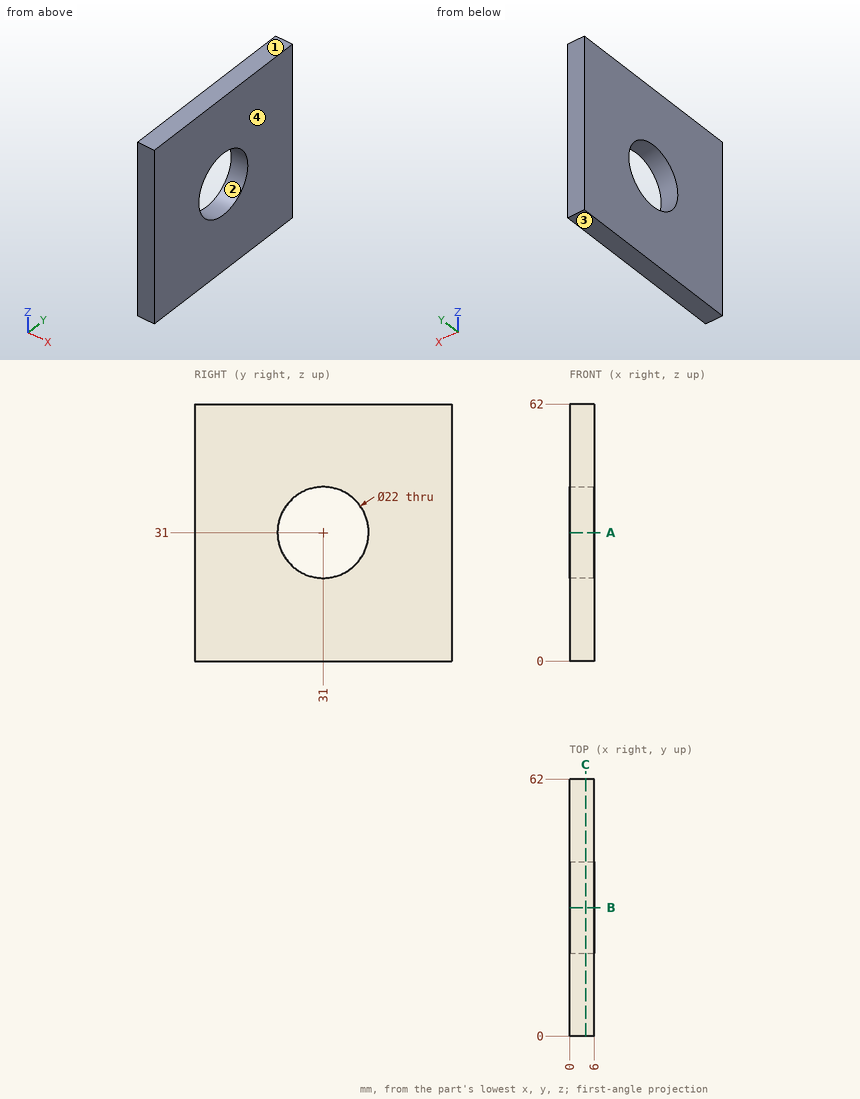
Check sheet for the drawn part. Datum: minimum x, y, z corner. Units: mm. Round coordinates to 2 decimals unless told otherwise and drop trailing zeros. Order: outer loops, then holes, each group sorted by start corner. A loop starts at its lowest first (then second) coordinate and runs counter-clockwise, first axis right, second up.
1) Section check A-A (z = 31). Record the boundary of the cut face in (x, y).
2) Section check C-C (x = 3.85). Record the boundary of the cut face in (y, z).
3) Mould release check, pull along Z, two halves, no side actions. Record for the marked faces 1, 2, 3 and 4: +Z half, -Z half, draft (parallel to the pull), parting line (faces both ways), or undercut.
4) Scan lines: line 1 (Z direction, x = 2.05, y = 30.5); line 2 (Y direction, x = 2.5, z = 31); line 3 (Y direction, x = 1.7, z = 21.5). Record each from-to range of solid material in increasing order.
Result:
1. outline: (0, 0) - (6, 0) - (6, 20) - (0, 20) - close; (0, 42) - (6, 42) - (6, 62) - (0, 62) - close
2. outline: (0, 0) - (62, 0) - (62, 62) - (0, 62) - close; hole circle Ø22 at (31, 31)
3. face 1: +Z half
3. face 2: undercut
3. face 3: -Z half
3. face 4: draft
4. line 1: z = 0 to 20.01, 41.99 to 62
4. line 2: y = 0 to 20, 42 to 62
4. line 3: y = 0 to 25.45, 36.55 to 62
